```python
from build123d import *

# Parameters (mm, degrees)
SKETCH_2_R          = 4.050000000000024
EXTRUDE_1_DEPTH     = 50
CUT_EXTRUDE_1_DEPTH = 100
CUT_EXTRUDE_2_DEPTH = 100
SKETCH_7_R          = 4.050000000000008
CUT_EXTRUDE_3_DEPTH = 100
CUT_EXTRUDE_6_DEPTH = 20
CUT_EXTRUDE_7_DEPTH = 20
CUT_EXTRUDE_8_DEPTH = 20
FILLET_1_R          = 6
FILLET_2_R          = 2
FILLET_3_R          = 6
FILLET_4_R          = 6
SKETCH_13_R         = 9.049999999999946
CUT_EXTRUDE_9_DEPTH = 2


with BuildPart() as part:
    # ｽｹｯﾁ2 → ﾎﾞｽ - 押し出し1 (new body)
    with BuildSketch(Plane(origin=(-3.9916e-13, 32.90329120575703, 627.8321969731651), x_dir=(-1, -3e-17, -6.3e-16), z_dir=(0, -0.05233595624294474, -0.9986295347545739))):
        Polygon((-697.0422820628135, 364.8089319187604), (-700.5932035956617, 324.9668567184454), (-636.3478573351539, 319.2409957467275), (-632.7969358023056, 359.08307094704253), align=None)
        with Locations(Location((-644.2839023988065, 340.0275704705168, 0), (0, 0, 90))):
            Circle(SKETCH_2_R, mode=Mode.SUBTRACT)
        with Locations(Location((-689.106236999161, 344.02235719497116, 0), (0, 0, 90))):
            Circle(SKETCH_2_R, mode=Mode.SUBTRACT)
    extrude(amount=EXTRUDE_1_DEPTH)

    # ｽｹｯﾁ5 → ｶｯﾄ - 押し出し1 (cut)
    with BuildSketch(Plane(origin=(723.8064708248907, 64.42078199043551, -3.3761501237952602), x_dir=(-0.004627728743617884, -0.0004118806842991107, -0.9999892071822463), z_dir=(0.9960518800078746, 0.08865137795745748, -0.004646021849131346))):
        Polygon((-608.1434669406992, 296.09511014614947), (-567.6985342683519, 293.98384959158335), (-567.3857549269345, 299.9756914689684), (-597.8442844703076, 301.56565312117255), (-596.645296994875, 324.5343803178144), (-566.186767451502, 322.9444186656103), (-565.8739881100848, 328.9362605429951), (-606.3189207824322, 331.0475210975612), (-626.0453368448235, 332.0772571204365), (-625.4050029902406, 344.3439854408341), (-551.5560275003857, 340.4890048871531), (-554.6576307812425, 281.07230447123857), (-628.5066062710979, 284.92728502491957), (-628.5066062710974, 296.97977053027586), align=None)
    extrude(amount=-CUT_EXTRUDE_1_DEPTH, mode=Mode.SUBTRACT)

    # ｽｹｯﾁ6 → ｶｯﾄ - 押し出し2 (cut)
    with BuildSketch(Plane(origin=(723.8064708248907, 64.42078199043551, -3.3761501237952602), x_dir=(-0.004627728743617884, -0.0004118806842991107, -0.9999892071822463), z_dir=(0.9960518800078746, 0.08865137795745748, -0.004646021849131346))):
        Polygon((-606.3189207824322, 331.04752109756123), (-608.1434669406992, 296.0951101461494), (-619.732969083748, 290.9532658931082), (-617.724208131906, 336.87839675393917), align=None)
    extrude(amount=-CUT_EXTRUDE_2_DEPTH, mode=Mode.SUBTRACT)

    # ｽｹｯﾁ7 → ｶｯﾄ - 押し出し3 (cut)
    with BuildSketch(Plane(origin=(-26.542256166274278, 297.4014749020998, -15.586150855120477), x_dir=(0.9960518800078747, 0.0886513779574575, -0.004646021849131969), z_dir=(-0.0887730383212076, 0.9946868255236824, -0.05212932760779488))):
        with Locations(Location((694.4254727867873, -591.2519877036084, 0), (0, 0, 179.733439165))):
            Circle(SKETCH_7_R)
    extrude(amount=-CUT_EXTRUDE_3_DEPTH, mode=Mode.SUBTRACT)

    # ｽｹｯﾁ8 → ｶｯﾄ - 押し出し6 (cut)
    with BuildSketch(Plane(origin=(-26.542256166274278, 297.4014749020998, -15.586150855120477), x_dir=(0.9960518800078747, 0.0886513779574575, -0.004646021849131969), z_dir=(-0.0887730383212076, 0.9946868255236824, -0.05212932760779488))):
        with BuildLine():
            Line((653.0837968072778, -612.7519877036083), (685.4254727867873, -612.7519877036083))
            Line((685.4254727867873, -612.7519877036083), (685.4254727867873, -591.2626120432828))
            ThreePointArc((685.4254727867873, -591.2626120432828), (694.420160616025, -582.2519830004186), (703.4254727867874, -591.2519877036085))
            Line((703.4254727867874, -591.2519877036085), (703.4254727867874, -612.7519877036083))
            Line((703.4254727867874, -612.7519877036083), (732.6544524188718, -612.7519877036083))
            Line((732.6544524188718, -612.7519877036083), (732.6544524188718, -571.4472878962366))
            Line((732.6544524188718, -571.4472878962366), (653.0837968072778, -571.4472878962366))
            Line((653.0837968072778, -571.4472878962366), (653.0837968072778, -612.7519877036083))
        make_face()
    extrude(amount=-CUT_EXTRUDE_6_DEPTH, mode=Mode.SUBTRACT)

    # ｽｹｯﾁ9 → ｶｯﾄ - 押し出し7 (cut)
    with BuildSketch(Plane(origin=(-23.96783805495928, 268.5555569619133, -14.074400354494276), x_dir=(0.9960518800078746, 0.08865137795745749, -0.0046460218491326), z_dir=(-0.08877303832120763, 0.994686825523682, -0.052129327607802006))):
        with BuildLine():
            Line((701.0201444957777, -585.1274220005872), (726.6754727867866, -612.7519877036101))
            Line((726.6754727867866, -612.7519877036101), (726.6754727867866, -582.25198770361))
            Line((726.6754727867866, -582.25198770361), (694.4254732410474, -582.25198770361))
            ThreePointArc((694.4254732410474, -582.2519877036095), (698.0226182987518, -583.0021062398702), (701.0201444957777, -585.1274220005872))
        make_face()
        with BuildLine():
            ThreePointArc((687.8308010777955, -585.1274220005871), (690.8283276912211, -583.0021060583099), (694.4254732410474, -582.2519877036095))
            Line((694.4254732410474, -582.25198770361), (662.1754727867867, -582.25198770361))
            Line((662.1754727867867, -582.25198770361), (662.1754727867866, -612.7519877036101))
            Line((662.1754727867866, -612.7519877036101), (687.8308010777955, -585.1274220005871))
        make_face()
    extrude(amount=-CUT_EXTRUDE_7_DEPTH, mode=Mode.SUBTRACT)

    # ｽｹｯﾁ10 → ｶｯﾄ - 押し出し8 (cut)
    with BuildSketch(Plane(origin=(-4.2186e-13, 32.06896121623387, 611.9122324003949), x_dir=(-1, -4e-17, -7.1e-16), z_dir=(0, -0.05233595624294566, -0.9986295347545738))):
        Polygon((-674.1060084484338, 360.25482907777223), (-697.885625926865, 355.3464390586851), (-697.2642146586165, 362.31880221874025), align=None)
        Polygon((-656.177074608292, 358.65691438799047), (-633.6427427973452, 349.59294124702217), (-633.0188683981086, 356.5929412470222), align=None)
    extrude(amount=-CUT_EXTRUDE_8_DEPTH, mode=Mode.SUBTRACT)

    # ﾌｨﾚｯﾄ1
    fillet_1_edges = [part.edges().sort_by_distance(p)[0] for p in [
        (700.3712709998582, 359.33885899665444, 599.767605561525),
        (636.1259247393505, 353.62084511839845, 600.0672739707941),
        (697.8856259268646, 387.19009011131783, 598.3079843885063),
        (633.6427427973448, 381.4444772684454, 598.6090991982213),
    ]]
    fillet(fillet_1_edges, radius=FILLET_1_R)

    # ﾌｨﾚｯﾄ2
    # the kernel refuses this fillet: 2 mm, written as the material it adds along each edge
    with BuildSketch(Plane(origin=(699.838632769931, 365.045300168582, 594.461681922105), x_dir=(-0.08877303832120755, 0.9946868255236814, -0.052129327607815884), z_dir=(-0.9960518800078746, -0.08865137795745748, 0.004646021849131346))) as fillet_2_piece_1_section:
        with BuildLine():
            CenterArc((FILLET_2_R, FILLET_2_R), FILLET_2_R, 180.00000000000324, 89.99999999999625)
            Line((2.78e-15, FILLET_2_R), (0, 0))
            Line((0, 0), (FILLET_2_R, 0))
        make_face()
    fillet_2_piece_1 = extrude(amount=64.49999999999983, mode=Mode.PRIVATE)
    fillet_2_piece_1 = split(fillet_2_piece_1, bisect_by=Plane(origin=(684.700257312396, 363.3009068359351, 578.2094916382387), z_dir=(-0.7298483504195092, -0.029343525726524503, 0.6829790208255727)), keep=Keep.TOP, mode=Mode.PRIVATE)
    fillet_2_piece_1 = split(fillet_2_piece_1, bisect_by=Plane(origin=(650.6507062336964, 360.2704024189458, 578.3683136457086), z_dir=(0.7298483504195105, 0.10057352631328549, 0.6761703566371646)), keep=Keep.TOP, mode=Mode.PRIVATE)
    add(fillet_2_piece_1)

    # ﾌｨﾚｯﾄ3
    fillet_3_edges = [part.edges().sort_by_distance(p)[0] for p in [
        (665.1415415283625, 391.55557073207024, 603.0860609736587),
    ]]
    fillet(fillet_3_edges, radius=FILLET_3_R)

    # ﾌｨﾚｯﾄ4
    fillet_4_edges = [part.edges().sort_by_distance(p)[0] for p in [
        (665.6741797582897, 385.06409021649864, 593.4125415917601),
        (656.4433937232551, 387.2502882914526, 593.2979678055787),
        (674.372327563397, 388.84601309468684, 593.2143394122943),
    ]]
    fillet(fillet_4_edges, radius=FILLET_4_R)

    # ｽｹｯﾁ13 → ｶｯﾄ - 押し出し9 (cut)
    with BuildSketch(Plane(origin=(-4.2186e-13, 32.06896121623387, 611.9122324003949), x_dir=(-1, -4e-17, -7e-16), z_dir=(0, -0.05233595624294553, -0.9986295347545739))):
        with Locations(Location((-689.106236999161, 344.02235719497077, 0), (0, 0, 90))):
            Circle(SKETCH_13_R)
        with Locations(Location((-644.2839023988065, 340.02757047051637, 0), (0, 0, 90))):
            Circle(SKETCH_13_R)
    extrude(amount=-CUT_EXTRUDE_9_DEPTH, mode=Mode.SUBTRACT)


solid = part.part
```
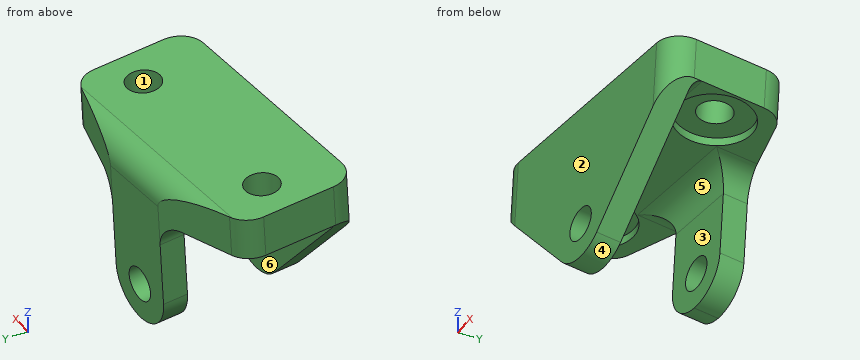
Design review of the part built by this model. Coordinates are the model's own, in mm. Face numbers are marked on the shaded views. A direction names the side the tool comes from. Give positions to 0.01 mm unless a question says otherwise; leave off trailing zeros. Order: outer loops, then holes, each group sorted by start corner. A loop starts at its lowest first (then second) coordinate and runs counter-clockwise, first axis right, second up. Notation, with made-up numbers: (-23, -7) -> (-5, -7) arc R17 ccw to (-5, -2) -> close; hole circle Ø6 at (16.5, 69.5). An arc over 180 degrees is marked (long way). Write each question's results on one line, items separated by ' | '. Start each with the question number.
Q1. Mouldability with a two-part tool opening along Z and no side actions: class the marked faces 1, 2 and 3 as +Z half, -Z half, draft (parallel to the pull), parting line (faces both ways), or undercut.
Q2. Add section B-B on x = 669. State how many separate pieces and enclosed holes the cut face has, and give its area (3 significant figures).
Q3. Wall thickness on L1, parallel to Y at x = 661, z = 588; L2, parallel to Y at x = 671, z = 567; L3, parallel to Z at x = 657, y = 369: over which ranges is each line inside the solid? List them lowest first. Write a range as from..to.
Q4. Machinability: for the marked faces 4, 5 and 6, which of the approach directions +Z, -Z, +X, -X, +Y, -Y give a long, thin tool a straight path to every point of the face, cutting with its end or side? Answer none if there is none.
Q5. Add section A-A on z = 584.5. Give the boundary of the cut face in (x, y).
Q6. For pin 1 (6 mm diameter, centred on x = 656, y = 369, fed in from +Z); pin 2 (12 mm diameter, centred on x = 660, z = 593, fed in from +Y); pin 3 (2 mm diameter, centred on x = 692, z = 588, fed in from +Y), all flat-tipped, find the tip position at first contact; note any pin that passes through.
Found:
1) face 1: parting line | face 2: +Z half | face 3: undercut
2) separate pieces: 3 | enclosed holes: 0 | area: 646 mm2
3) L1: y = 355.21..361.24, 384.34..390.4 | L2: y = 355..361.03, 384.16..390.19 | L3: z = 594.25..604.27
4) face 4: -Z | face 5: +X | face 6: -Z, -X
5) outline: (645.06, 359.63) -> (645.88, 353.68) -> (690.81, 357.69) -> (690.57, 363.7) -> close; (656.18, 389.78) -> (656.71, 383.8) -> (674.64, 385.4) -> (674.11, 391.38) -> close
6) pin 1: stops at z = 604.43 | pin 2: stops at y = 391.19 | pin 3: stops at y = 364.11
